Could you check a few things on this drawing? It's one solid part, dimensions in mm from its lowest x, y, z. Give positions to 0.01 mm unless a question says otherwise; leave off trailing zeros. Loops run counter-clockwise (first coordinate to the right, second up) from the corner with the lowest first, then second, coordinate; pieces in that order, holes last. Notation, with made-up numbers: (-23.5, 13.25) - (28.5, 13.25) arc R16 ccw to (28.5, 17.25) - close; hole circle Ø5 at (-24.5, 31). An arc over 180 degrees is marked (long way). Use a Markdown table: item, result.
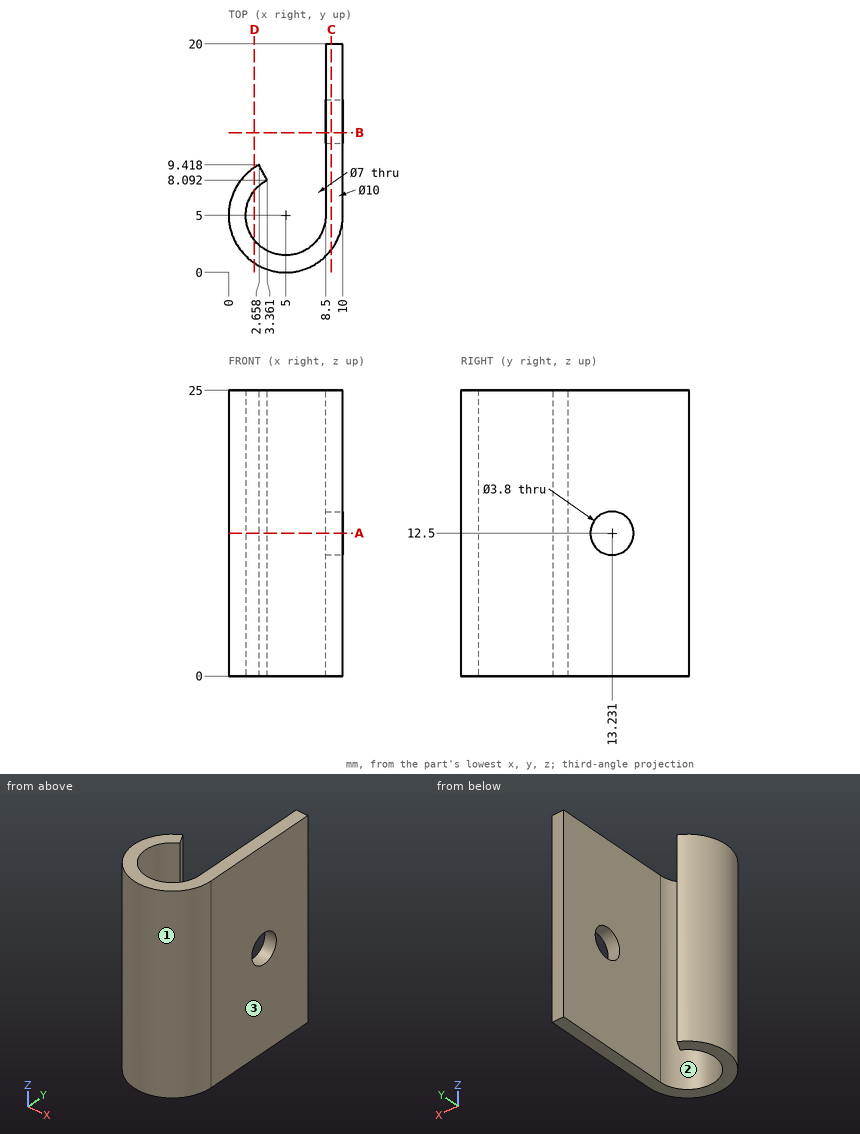
(1) Suppose I cut it at D-D on x = 2.25. Write out the boundary of the cut face in (y, z) (1 decimal).
A:
| item | result |
|---|---|
| outline | (0.8, 0) - (2.8, 0) - (2.8, 25) - (0.8, 25) - close; (7.2, 0) - (9.2, 0) - (9.2, 25) - (7.2, 25) - close |
(2) Suppose I cut it at C-C on x = 9. Write out the boundary of the cut face in (y, z), plus the area to 3 significant figures.
A:
| item | result |
|---|---|
| outline | (2, 0) - (20, 0) - (20, 25) - (2, 25) - close; hole circle Ø3.8 at (13.23, 12.5) |
| area | 439 mm2 |
(3) If I drill on line 1 (X direction, y = 5, z = 9.25); line 2 (X direction, y = 8.25, z = 7.25); line 3 (X direction, y = 12.5, z = 3), over which ranges is the centre line in solid material (lowest first)?
A:
| item | result |
|---|---|
| line 1 | 0 to 1.5, 8.5 to 10 |
| line 2 | 1.2 to 3.28, 8.5 to 10 |
| line 3 | 8.5 to 10 |
(4) Will these pins go through, and if not, where does the flat tip stop? pin 1 (1.5 mm diameter, centred on y = 14, z = 10.5, fed in from -X); pin 2 (4 mm diameter, centred on x = 1.5, z = 16, fed in from +Y); pin 3 (7.5 mm diameter, centred on y = 12, z = 13.5, fed in from -X); pin 4 (2 mm diameter, centred on x = 6.5, y = 10.5, fed in from -Z).
A:
| item | result |
|---|---|
| pin 1 | x = 8.5 |
| pin 2 | y = 9.42 |
| pin 3 | x = 1.2 |
| pin 4 | through |
(5) We'd pull the mould along X, two halves only. Please class the marked faces 1, 2 and 3: pulls with the +X half, pulls with the -X half, needs draft (parallel to the pull), parting line crosses it, or undercut.
A:
| item | result |
|---|---|
| face 1 | parting line crosses it |
| face 2 | undercut |
| face 3 | pulls with the +X half |
(6) Suppose I cut it at B-B on y = 12.25. Write out the boundary of the cut face in (x, z).
A:
| item | result |
|---|---|
| outline | (8.5, 0) - (10, 0) - (10, 10.87) - (8.5, 10.87) - close; (8.5, 14.13) - (10, 14.13) - (10, 25) - (8.5, 25) - close |
(7) Suppose I cut it at A-A on z = 12.5. Write out the boundary of the cut face in (x, y).
A:
| item | result |
|---|---|
| outline | (2.66, 9.42) arc R5 ccw (long way) to (10, 5) - (10, 11.33) - (8.5, 11.33) - (8.5, 5) arc R3.5 cw (long way) to (3.36, 8.09) - close; (8.5, 15.13) - (10, 15.13) - (10, 20) - (8.5, 20) - close |
